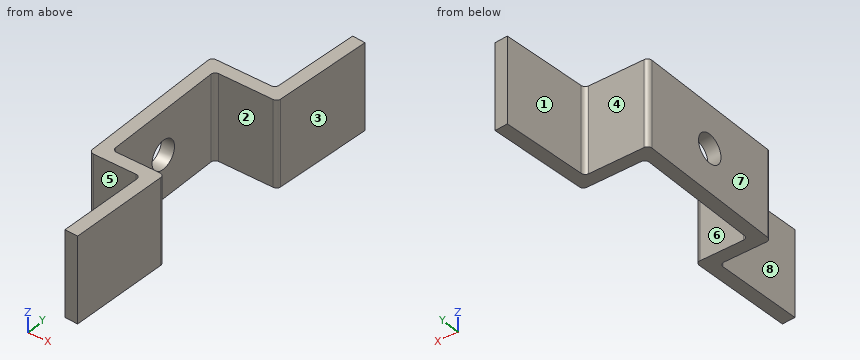
```python
from build123d import *

# Parameters (mm, degrees)
EXTRUDE_1_DEPTH      = 10
EXTRUDE_1_DEPTH_BACK = 10
HOLE_WIZARD_M61_D    = 6.6


with BuildPart() as part:
    # Эскиз1 → Бобышка-Вытянуть1 (new, two sides: drawn at the far end of the back side and taken through both)
    with BuildSketch(Plane.XY.offset(-EXTRUDE_1_DEPTH_BACK)):
        with BuildLine():
            Line((0, 17), (0, -17))
            ThreePointArc((0, -17), (0.292893219, -17.707106781), (1, -18))
            Line((1, -18), (10.821545488, -18))
            ThreePointArc((10.821545488, -18), (11.54390945, -18.308486944), (11.820593709, -19.043619387))
            Line((11.820593709, -19.043619387), (10.948205962, -39.024583819))
            Line((10.948205962, -39.024583819), (13.945350627, -39.155441981))
            Line((13.945350627, -39.155441981), (14.954434594, -16.043619387))
            ThreePointArc((14.954434594, -16.043619387), (14.677750334, -15.308486944), (13.955386372, -15))
            Line((13.955386372, -15), (4, -15))
            ThreePointArc((4, -15), (3.292893219, -14.707106781), (3, -14))
            Line((3, -14), (3, 14))
            ThreePointArc((3, 14), (3.292893219, 14.707106781), (4, 15))
            Line((4, 15), (16.567484914, 15))
            ThreePointArc((16.567484914, 15), (17.249483274, 15.268646298), (17.565048964, 15.930243526))
            Line((17.565048964, 15.930243526), (19.155325331, 38.67225511))
            Line((19.155325331, 38.67225511), (16.162633181, 38.881524531))
            Line((16.162633181, 38.881524531), (14.767503706, 18.930243526))
            ThreePointArc((14.767503706, 18.930243526), (14.451938016, 18.268646298), (13.769939655, 18))
            Line((13.769939655, 18), (1, 18))
            ThreePointArc((1, 18), (0.292893219, 17.707106781), (0, 17))
        make_face()
    extrude(amount=EXTRUDE_1_DEPTH + EXTRUDE_1_DEPTH_BACK)

    # Отверстие с зазором M61 (through all)
    with Locations(Plane(origin=(0, 0, 0), x_dir=(0, -1, 0), z_dir=(-1, 0, 0))):
        with Locations((0, 0)):
            Hole(HOLE_WIZARD_M61_D / 2)


solid = part.part
```
Check sheet for the modelled part. Datum: model origin and axes. Units: mm. Face numbers are marked on the shaded views. A direction names the side the tool comes from. Round coordinates to 2 decimals unless told otherwise and drop trailing zeros. Loops run counter-clockwise (first coordinate to the right, second up) from the corner with the lowest first, then second, coordinate; pieces in that order, holes last. Notation, with made-up numbers: (-3.75, 45) - (48.25, 45) arc R15 ccw to (48.25, 57) - close; hole circle Ø11 at (-36, 71). An arc over 180 degrees is marked (long way). Write item = value, one per line. Start each with the question number.
Q1. Access from +Z, -Z, +X, -X, +Y, -Y to the whole of each face (thin tool, end or side, straight path). Record for the marked faces 4, 5, 6, 7 and 8.
Q2. Section check C-C (z = 0). Record the boundary of the cut face in (x, y), plus the area to 3 significant figures.
Q3. Section check A-A (y = 0). Record the boundary of the cut face in (x, z), plus the area to 3 significant figures.
Q4. Release check for a two-part mould opening along Y. For the marked faces 1, 2 and 3 record: pulls with the +Y half, pulls with the -Y half, needs draft (parallel to the pull), parting line crosses it, or undercut.
Q5. Depth check by flat-ended pin: P1, Ø4, axis at x = 17, y = -30, coming from the -Z side; P2, Ø2, axis at x = 6, z = 7.5, coming from the +Y side; P3, Ø1.5, axis at y = -30.5, z = 0.5, coming from the +X side; P4, Ø1, axis at y = 30, z = -2.5, coming from the -X side. Enter the tip coordinate at first touch or a pass-through.
Q6. Section check D-D (z = 5.75). Record the boundary of the cut face in (x, y), plus the area to 3 significant figures.
Q7. Section check B-B (x = 9.5). Record the boundary of the cut face in (y, z).
Q8. Thickness scan on L1, parallel to Y at x = 4.5, z = -0.25; L2, parallel to Y at x = 2.5, z = -6.25; L3, parallel to Z at x = 1.5, y = -0.5. Record the ranges inside material, lowest first.
Derived:
q1.face_4 = +Z, -Z, -X, +Y
q1.face_5 = +Z, -Z, -X, -Y
q1.face_6 = +Z, -Z, +X
q1.face_7 = +Z, -Z, -X, +Y, -Y
q1.face_8 = +Z, -Z, -X
q2.outline = (0, -17) arc R1 ccw to (1, -18) - (10.82, -18) arc R1 cw to (11.82, -19.04) - (10.95, -39.02) - (13.95, -39.16) - (14.95, -16.04) arc R1 ccw to (13.96, -15) - (4, -15) arc R1 cw to (3, -14) - (3, -3.3) - (0, -3.3) - close; (0, 3.3) - (3, 3.3) - (3, 14) arc R1 cw to (4, 15) - (16.57, 15) arc R1 ccw to (17.57, 15.93) - (19.16, 38.67) - (16.16, 38.88) - (14.77, 18.93) arc R1 cw to (13.77, 18) - (1, 18) arc R1 ccw to (0, 17) - close
q2.area = 294 mm^2
q3.outline = (0, -10) - (3, -10) - (3, -3.3) - (0, -3.3) - close; (0, 3.3) - (3, 3.3) - (3, 10) - (0, 10) - close
q3.area = 40.2 mm^2
q4.face_1 = pulls with the +Y half
q4.face_2 = undercut
q4.face_3 = pulls with the -Y half
q5.P1 = through
q5.P2 = 18
q5.P3 = 14.36
q5.P4 = 15.51
q6.outline = (0, -17) arc R1 ccw to (1, -18) - (10.82, -18) arc R1 cw to (11.82, -19.04) - (10.95, -39.02) - (13.95, -39.16) - (14.95, -16.04) arc R1 ccw to (13.96, -15) - (4, -15) arc R1 cw to (3, -14) - (3, 14) arc R1 cw to (4, 15) - (16.57, 15) arc R1 ccw to (17.57, 15.93) - (19.16, 38.67) - (16.16, 38.88) - (14.77, 18.93) arc R1 cw to (13.77, 18) - (1, 18) arc R1 ccw to (0, 17) - close
q6.area = 313 mm^2
q7.outline = (-18, -10) - (-15, -10) - (-15, 10) - (-18, 10) - close; (15, -10) - (18, -10) - (18, 10) - (15, 10) - close
q8.L1 = -18 to -15, 15 to 18
q8.L2 = -18 to 18
q8.L3 = -10 to -3.26, 3.26 to 10
